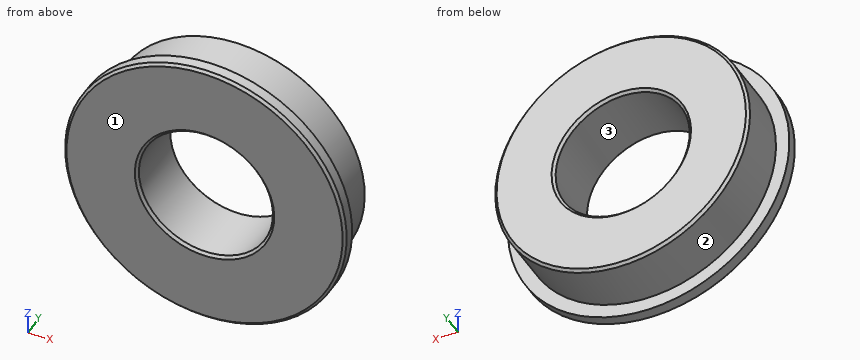
from build123d import *

# Parameters (mm, degrees)
SKETCH_1_R      = 9.5
SKETCH_1_R_2    = 5
EXTRUDE_1_DEPTH = 5
SKETCH_2_R      = 10.5
SKETCH_2_R_2    = 9.5
EXTRUDE_2_DEPTH = 1
CHAMFER_1_SIZE  = 0.2


with BuildPart() as part:
    # 草图1 → 凸台-拉伸1 (new body)
    with BuildSketch(Plane(origin=(0, 0, 0), x_dir=(1, 0, 0), z_dir=(0, 1, 0))):
        with Locations(Location((0, 0, 0), (0, 0, 270))):
            Circle(SKETCH_1_R)
        with Locations(Location((0, 0, 0), (0, 0, 270))):
            Circle(SKETCH_1_R_2, mode=Mode.SUBTRACT)
    extrude(amount=EXTRUDE_1_DEPTH)

    # 草图2 → 凸台-拉伸2 (add)
    with BuildSketch(Plane.XZ):
        with Locations(Location((0, 0, 0), (0, 0, 270))):
            Circle(SKETCH_2_R)
        with Locations(Location((0, 0, 0), (0, 0, 270))):
            Circle(SKETCH_2_R_2, mode=Mode.SUBTRACT)
    extrude(amount=-EXTRUDE_2_DEPTH)

    # 倒角1
    chamfer_1_edges = [part.edges().sort_by_distance(p)[0] for p in [
        (0, 0, 10.5),
        (0, 5, -9.5),
        (0, 0, -5),
        (0, 5, -5),
    ]]
    chamfer(chamfer_1_edges, length=CHAMFER_1_SIZE)


solid = part.part
Geometry check sheet. Reference: the model listing, model coordinates, mm. Face numbers are marked on the shaded views. Give positions to 0.01 mm unless a question says otherwise; leave off trailing zeros. Order: outer loops, then holes, each group sorted by start corner. A loop starts at its lowest first (then second) coordinate and runs counter-clockwise, first axis right, second up. Notation, with made-up numbers: (72, 89) - (130, 89) arc R20 cw to (130, 93) - close; hole circle Ø11 at (32, -28.75). An arc over 180 degrees is marked (long way). Use one line per item in the form item = value.
1) Depth check by flat-ended pin: pin 1 Ø1.5 at (x, z) = (2, -3.5) entering from +Y; pin 2 Ø3 at (x, y) = (-7, 1) entering from -Z; pin 3 Ø3 at (y, z) = (2, 4) entering from +X; pin 4 Ø1 at (x, y) = (2, 4) entering from +Z. Enter the tip coordinate at first touch or a pass-through.
Working result:
pin_1 = through
pin_2 = -8.94
pin_3 = 10.1
pin_4 = 9.38
2) Draft check along X on the marked faces 1, 2 and 3. Enter one of: released by +X, released by -X, zero draft, split by the parting line, or undercut.
Working result:
face_1 = zero draft
face_2 = split by the parting line
face_3 = undercut
3) Sectioned sample at C-C (y = 1.4). Record the boundary of the cut face in (x, z), and give its area (3 significant figures).
Working result:
outline = circle Ø19 at (0, 0); hole circle Ø10 at (0, 0)
area = 205 mm^2
4) Sectioned sample at A-A (z = 0). Record the boundary of the cut face in (x, y), and give its area (3 significant figures).
Working result:
outline = (-10.5, 0.2) - (-10.3, 0) - (-5.2, 0) - (-5, 0.2) - (-5, 4.8) - (-5.2, 5) - (-9.3, 5) - (-9.5, 4.8) - (-9.5, 1) - (-10.5, 1) - close; (5, 0.2) - (5.2, 0) - (10.3, 0) - (10.5, 0.2) - (10.5, 1) - (9.5, 1) - (9.5, 4.8) - (9.3, 5) - (5.2, 5) - (5, 4.8) - close
area = 46.8 mm^2
5) Material ranges on probe 1 along X at (y, z) = (3.6, 0); probe 2 along Z at (x, y) = (0.25, 2.75); probe 3 along Z at (x, y) = (3, 4.6), recorded low to high. Write a range as from..to.
Working result:
probe_1 = -9.5..-5, 5..9.5
probe_2 = -9.5..-4.99, 4.99..9.5
probe_3 = -9.01..-4, 4..9.01
6) Sectioned sample at B-B (x = 0). Record the boundary of the cut face in (y, z), and give its area (3 significant figures).
Working result:
outline = (0, -10.3) - (0.2, -10.5) - (1, -10.5) - (1, -9.5) - (4.8, -9.5) - (5, -9.3) - (5, -5.2) - (4.8, -5) - (0.2, -5) - (0, -5.2) - close; (0, 5.2) - (0.2, 5) - (4.8, 5) - (5, 5.2) - (5, 9.3) - (4.8, 9.5) - (1, 9.5) - (1, 10.5) - (0.2, 10.5) - (0, 10.3) - close
area = 46.8 mm^2
